Check sheet for the modelled part. Datum: model origin and axes. Units: mm. Face numbers are marked on the shaded views. A direction names the side the tool comes from. Give positions to 0.01 mm unless a question says otherwise; leave off trailing zeros. Write each loop counter-clockwise with the first axis right and the second up, starting at its lowest first coordinate (ties: lowest second). Pieces come first, ordered by that corner, then holes. Notation, with made-up numbers: M 23,-12 L 28,-12 A7 cw 28,-3 Z; hole C -3,1.25 d9. An arc over 180 degrees is marked long. Write item = value, one per line. Start each with the question number.
1) Sectioned sample at B-B, the plane y = -79.5. Record the cut outline in (x, z).
2) Draft check along X on the marked faces 4, 5 and 6. Enter one of: pulls with the +X half, pulls with the -X half, needs draft (parallel to the pull), parting line crosses it, or undercut.
3) Set-up check for the marked faces 1, 2 and 3: record each of +Z, -Z, +X, -X, +Y, -Y from which the full face is reachable in a straight line by a thin tool's end or side.
4) Scan lines: L1, parallel to X at y = -76, z = 33; L2, parallel to Y at x = 56, z = 12; L3, parallel to Y at x = 1.5, z = 23. Record each from-to range of solid material in increasing order.
5) Sectioned sample at D-D, the plane x = -26. Record the cut outline in (y, z).
6) Sectioned sample at A-A, the plane z = 8. Record the cut outline in (x, y).
7) Sectioned sample at C-C, the plane z = 23.5. Record the cut outline in (x, y).
8) Gauge pin test, flat ends, axial feed: pin 1 (4 mm diameter, centred on y = -11.5, z = 28, fed in from -X); pin 2 (4.5 mm diameter, centred on x = -74, y = -105, fed in from +Z); pin 3 (4 mm diameter, centred on x = 71.81, y = -18.86, fed in from -Z); pin 4 (10 mm diameter, centred on x = 69.5, z = 39, fed in from -Y). Record the tip position at first contact, or that the pin passes through.
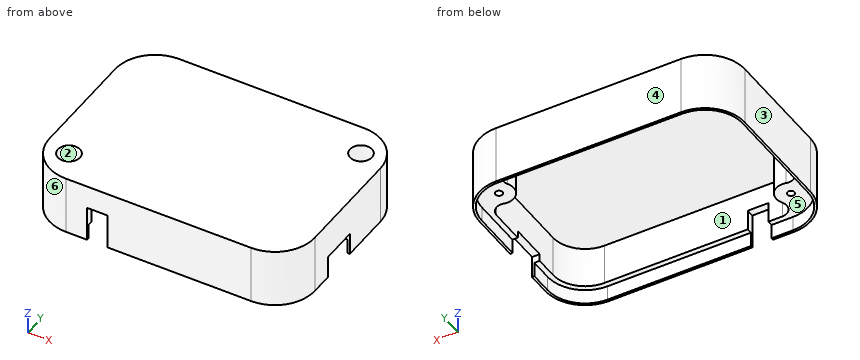
from build123d import *

# Parameters (mm, degrees)
PAD002_DEPTH    = 30
PAD003_DEPTH    = 10
POCKET011_DEPTH = 10
POCKET012_DEPTH = 28
PAD004_DEPTH    = 28
SKETCH018_R     = 2.4
POCKET013_DEPTH = 30.001
SKETCH019_R     = 7.5
POCKET014_DEPTH = 12
SKETCH020_W     = 14
SKETCH020_H     = 40
POCKET015_DEPTH = 5.201
SKETCH021_W     = 25
SKETCH021_H     = 30
POCKET016_DEPTH = 10


with BuildPart() as part:
    # Sketch013 (on Face25 of Binder) → Pad002 (new body)
    with BuildSketch(Plane.XY.offset(15)):
        with BuildLine():
            Line((-64.5, 2.2), (61.5, 2.2))
            ThreePointArc((88.7, -25), (80.733304, -5.766696), (61.5, 2.2))
            Line((88.7, -25), (88.7, -100))
            ThreePointArc((61.5, -127.2), (80.733304, -119.233304), (88.7, -100))
            Line((-64.5, -127.2), (61.5, -127.2))
            ThreePointArc((-91.7, -100), (-83.733304, -119.233304), (-64.5, -127.2))
            Line((-91.7, -25), (-91.7, -100))
            ThreePointArc((-64.5, 2.2), (-83.733304, -5.766696), (-91.7, -25))
        make_face()
    extrude(amount=PAD002_DEPTH)

    # Sketch014 (on Face9 of Pad002) → Pad003 (join)
    with BuildSketch(Plane(origin=(0, 0, 15), x_dir=(1, 0, 0), z_dir=(0, 0, -1))):
        with BuildLine():
            Line((-64.5, 127.2), (61.5, 127.2))
            ThreePointArc((88.7, 100), (80.733304, 119.233304), (61.5, 127.2))
            Line((88.7, 25), (88.7, 100))
            ThreePointArc((61.5, -2.2), (80.733304, 5.766696), (88.7, 25))
            Line((-64.5, -2.2), (61.5, -2.2))
            ThreePointArc((-91.7, 25), (-83.733304, 5.766696), (-64.5, -2.2))
            Line((-91.7, 100), (-91.7, 25))
            ThreePointArc((-64.5, 127.2), (-83.733304, 119.233304), (-91.7, 100))
        make_face()
    extrude(amount=PAD003_DEPTH)

    # Sketch015 (on Face10 of Pad003) → Pocket011 (cut)
    with BuildSketch(Plane(origin=(0, 0, 5), x_dir=(1, 0, 0), z_dir=(0, 0, -1))):
        with BuildLine():
            Line((-64.5, 125.6), (61.5, 125.6))
            ThreePointArc((87.1, 100), (79.601934, 118.101934), (61.5, 125.6))
            Line((87.1, 100), (87.1, 25))
            ThreePointArc((61.5, -0.6), (79.601934, 6.898066), (87.1, 25))
            Line((-64.5, -0.6), (61.5, -0.6))
            ThreePointArc((-90.1, 25), (-82.601934, 6.898066), (-64.5, -0.6))
            Line((-90.1, 100), (-90.1, 25))
            ThreePointArc((-64.5, 125.6), (-82.601934, 118.101934), (-90.1, 100))
        make_face()
    extrude(amount=-POCKET011_DEPTH, mode=Mode.SUBTRACT)

    # Sketch016 (on Face27 of Pocket011) → Pocket012 (cut)
    with BuildSketch(Plane(origin=(0, 0, 15), x_dir=(1, 0, 0), z_dir=(0, 0, -1))):
        with BuildLine():
            Line((-64.5, 122), (61.5, 122))
            ThreePointArc((83.5, 100), (77.056349, 115.556349), (61.5, 122))
            Line((83.5, 100), (83.5, 25))
            ThreePointArc((61.5, 3), (77.056349, 9.443651), (83.5, 25))
            Line((-64.5, 3), (61.5, 3))
            ThreePointArc((-86.5, 25), (-80.056349, 9.443651), (-64.5, 3))
            Line((-86.5, 100), (-86.5, 25))
            ThreePointArc((-64.5, 122), (-80.056349, 115.556349), (-86.5, 100))
        make_face()
    extrude(amount=-POCKET012_DEPTH, mode=Mode.SUBTRACT)

    # Sketch017 (on Face36 of Pocket012) → Pad004 (join)
    with BuildSketch(Plane(origin=(0, 0, 43), x_dir=(1, 0, 0), z_dir=(0, 0, -1))):
        with BuildLine():
            ThreePointArc((-64.5, 122), (-80.056349, 115.556349), (-86.5, 100))
            Line((-86.5, 100), (-86.5, 89.146438))
            ThreePointArc((-77.204935, 96.428453), (-83.625311, 95.050377), (-86.5, 89.146438))
            ThreePointArc((-77.204935, 96.428453), (-66.894122, 100.029214), (-66.027044, 110.916203))
            ThreePointArc((-59.438691, 122), (-65.885724, 118.3322), (-66.027044, 110.916203))
            Line((-64.5, 122), (-59.438691, 122))
        make_face()
        with BuildLine():
            ThreePointArc((61.5, 3), (77.056349, 9.443651), (83.5, 25))
            Line((83.5, 35.853562), (83.5, 25))
            ThreePointArc((74.204935, 28.571547), (80.625311, 29.949623), (83.5, 35.853562))
            ThreePointArc((74.204935, 28.571547), (63.894122, 24.970786), (63.027044, 14.083797))
            ThreePointArc((56.438691, 3), (62.885724, 6.6678), (63.027044, 14.083797))
            Line((56.438691, 3), (61.5, 3))
        make_face()
    extrude(amount=PAD004_DEPTH)

    # Sketch018 (on Face28 of Pad004) → Pocket013 (cut, through all)
    with BuildSketch(Plane(origin=(0, 0, 15), x_dir=(1, 0, 0), z_dir=(0, 0, -1))):
        with Locations((-74.811515, 106.137806)):
            Circle(SKETCH018_R)
        with Locations((71.811515, 18.862194)):
            Circle(SKETCH018_R)
    extrude(amount=-POCKET013_DEPTH, mode=Mode.SUBTRACT)

    # Sketch019 (on Face5 of Pocket013) → Pocket014 (cut)
    with BuildSketch(Plane.XY.offset(45)):
        with Locations((71.811515, -18.862194)):
            Circle(SKETCH019_R)
        with Locations((-74.811515, -106.137806)):
            Circle(SKETCH019_R)
    extrude(amount=-POCKET014_DEPTH, mode=Mode.SUBTRACT)

    # Sketch020 (on Face35 of Pocket014) → Pocket015 (cut, through all)
    with BuildSketch(Plane(origin=(0, -122, 0), x_dir=(-1, 0, 0), z_dir=(0, 1, 0))):
        with Locations((43, 9)):
            Rectangle(SKETCH020_W, SKETCH020_H)
    extrude(amount=-POCKET015_DEPTH, mode=Mode.SUBTRACT)

    # Sketch021 (on Face11 of Pocket015) → Pocket016 (cut)
    with BuildSketch(Plane.YZ.offset(88.7)):
        with Locations((-72.5, 5)):
            Rectangle(SKETCH021_W, SKETCH021_H)
    extrude(amount=-POCKET016_DEPTH, mode=Mode.SUBTRACT)


solid = part.part
Data:
q1.outline = M -91.7,5 L -90.1,5 L -90.1,15 L -86.5,15 L -86.5,43 L 83.5,43 L 83.5,20 L 88.7,20 L 88.7,45 L -91.7,45 Z
q2.face_4 = needs draft
q2.face_5 = undercut
q2.face_6 = pulls with the -X half
q3.face_1 = -Z
q3.face_2 = +Z
q3.face_3 = +Z, -Z, -X, +Y, -Y
q4.L1 = -91.7 to -86.5, 83.5 to 88.7
q4.L2 = -127.2 to -125.6, 0.6 to 2.2
q4.L3 = -127.2 to -122, -3 to 2.2
q5.outline = M -127.2,5 L -125.6,5 L -125.6,15 L -122,15 L -122,43 L -3,43 L -3,15 L 0.6,15 L 0.6,5 L 2.2,5 L 2.2,45 L -127.2,45 Z
q6.outline = M -91.7,-100 A27.2 ccw -64.5,-127.2 L -50,-127.2 L -50,-125.6 L -64.5,-125.6 A25.6 cw -90.1,-100 L -90.1,-25 A25.6 cw -64.5,0.6 L 61.5,0.6 A25.6 cw 87.1,-25 L 87.1,-60 L 88.7,-60 L 88.7,-25 A27.2 ccw 61.5,2.2 L -64.5,2.2 A27.2 ccw -91.7,-25 Z; M -36,-127.2 L 61.5,-127.2 A27.2 ccw 88.7,-100 L 88.7,-85 L 87.1,-85 L 87.1,-100 A25.6 cw 61.5,-125.6 L -36,-125.6 Z
q7.outline = M -91.7,-100 A27.2 ccw -64.5,-127.2 L -50,-127.2 L -50,-122 L -59.44,-122 A7.5 cw -66.03,-110.92 A10 ccw -77.2,-96.43 A7.5 cw -86.5,-89.15 L -86.5,-25 A22 cw -64.5,-3 L 56.44,-3 A7.5 cw 63.03,-14.08 A10 ccw 74.2,-28.57 A7.5 cw 83.5,-35.85 L 83.5,-100 A22 cw 61.5,-122 L -36,-122 L -36,-127.2 L 61.5,-127.2 A27.2 ccw 88.7,-100 L 88.7,-25 A27.2 ccw 61.5,2.2 L -64.5,2.2 A27.2 ccw -91.7,-25 Z; hole C -74.81,-106.14 d4.8; hole C 71.81,-18.86 d4.8
q8.pin_1 = -89.15
q8.pin_2 = 33
q8.pin_3 = through
q8.pin_4 = -127.03
